from build123d import *

# Parameters (mm, degrees)
BOSS_EXTRUDE1_DEPTH  = 12
SKETCH2_R            = 1.6
CUT_EXTRUDE1_DEPTH   = 12
SKETCH3_R            = 3
CUT_EXTRUDE2_DEPTH   = 2
BOSS_EXTRUDE2_DEPTH  = 2
MIRROR2_COPY_1_DEPTH = 2
SKETCH5_W            = 40
SKETCH5_H            = 1
CUT_EXTRUDE3_DEPTH   = 20


with BuildPart() as part:
    # Sketch1 → Boss-Extrude1 (new body)
    with BuildSketch(Plane(origin=(0, 0, 0), x_dir=(1, 0, 0), z_dir=(0, 1, 0))):
        with BuildLine():
            Line((13, 0), (20, 0))
            Line((20, 0), (20, 5))
            Line((20, 5), (12, 5))
            ThreePointArc((12, 5), (12.747548784, 2.549509757), (13, 0))
        make_face()
        with BuildLine():
            Line((8, 0), (13, 0))
            ThreePointArc((13, 0), (12.747548784, 2.549509757), (12, 5))
            Line((12, 5), (6.244997998, 5))
            ThreePointArc((6.244997998, 5), (7.548509256, 2.649529771), (8, 0))
        make_face()
        with BuildLine():
            ThreePointArc((-12, 5), (-12.747548784, 2.549509757), (-13, 0))
            Line((-13, 0), (-8, 0))
            ThreePointArc((-8, 0), (-7.548509256, 2.649529771), (-6.244997998, 5))
            Line((-6.244997998, 5), (-12, 5))
        make_face()
        with BuildLine():
            Line((6.244997998, 5), (12, 5))
            ThreePointArc((12, 5), (0, 13), (-12, 5))
            Line((-12, 5), (-6.244997998, 5))
            ThreePointArc((-6.244997998, 5), (0, 8), (6.244997998, 5))
        make_face()
        with BuildLine():
            Line((-20, 0), (-13, 0))
            ThreePointArc((-13, 0), (-12.747548784, 2.549509757), (-12, 5))
            Line((-12, 5), (-20, 5))
            Line((-20, 5), (-20, 0))
        make_face()
    extrude(amount=BOSS_EXTRUDE1_DEPTH)

    # Sketch2 → Cut-Extrude1 (cut)
    with BuildSketch(Plane(origin=(0, 0, -5), x_dir=(-1, 0, 0), z_dir=(0, 0, -1))):
        with Locations((16, 6)):
            Circle(SKETCH2_R)
        with Locations((-16, 6)):
            Circle(SKETCH2_R)
    extrude(amount=-CUT_EXTRUDE1_DEPTH, mode=Mode.SUBTRACT)

    # Sketch3 → Cut-Extrude2 (cut)
    with BuildSketch(Plane(origin=(0, 0, -5), x_dir=(-1, 0, 0), z_dir=(0, 0, -1))):
        with Locations((16, 6)):
            Circle(SKETCH3_R)
        with Locations((-16, 6)):
            Circle(SKETCH3_R)
    extrude(amount=-CUT_EXTRUDE2_DEPTH, mode=Mode.SUBTRACT)

    # Sketch4 → Boss-Extrude2 (add)
    with BuildSketch(Plane(origin=(0, 12, 0), x_dir=(1, 0, 0), z_dir=(0, 1, 0))):
        Polygon((-20, 5), (-5.505882353, 11.776470588), (-3.437353346, 7.352116879), (-12, 5), align=None)
    boss_extrude2 = extrude(amount=-BOSS_EXTRUDE2_DEPTH)

    # Mirror1: Boss-Extrude2 across plane
    add(boss_extrude2.mirror(Plane(origin=(0, 0, 0), x_dir=(0, 0, 1), z_dir=(1, 0, 0))))

    # Mirror2: Boss-Extrude2 across plane
    add(boss_extrude2.mirror(Plane.ZX.offset(6)))

    # Mirror2 copy 1 sketch → Mirror2 copy 1 (add)
    with BuildSketch(Plane(origin=(0, 0, 0), x_dir=(-1, 0, 0), z_dir=(0, -1, 0))):
        Polygon((-20, 5), (-5.505882353, 11.776470588), (-3.437353346, 7.352116879), (-12, 5), align=None)
    extrude(amount=-MIRROR2_COPY_1_DEPTH)

    # Chamfer1
    # the kernel refuses this chamfer: 5 mm, written as the material it adds along each edge
    with BuildSketch(Plane(origin=(-12, 2, -5), x_dir=(0.5282334615554308, 0, -0.8490991756521539), z_dir=(0, 1, 0))) as chamfer1_piece_1_section:
        with BuildLine():
            Line((3.55102746, 0), (-2.413771098, 3.712725473))
            Line((-2.413771098, 3.712725473), (-2.498681015, 3.659902127))
            ThreePointArc((-2.498681015, 3.659902127), (-1.254288539, 1.826872841), (-0.084909918, -0.052823346))
            Line((-0.084909918, -0.052823346), (0.016102351, -0.098695057))
            ThreePointArc((0.016102351, -0.098695057), (1.773886736, 0.065687387), (3.541120329, -0.099508034))
            Line((3.541120329, -0.099508034), (3.55102746, 0))
        make_face()
    chamfer1_piece_1 = extrude(amount=8, mode=Mode.PRIVATE)
    chamfer1_piece_1 = chamfer1_piece_1 - Plane(origin=(-16, 6, -6.086552006), x_dir=(-1, 0, 0), z_dir=(0, 0, -1)) * Cylinder(3, 31, mode=Mode.PRIVATE)
    add(chamfer1_piece_1)
    with BuildSketch(Plane(origin=(12, 2, -5), x_dir=(0.9998009840016291, 0, 0.01994974659924107), z_dir=(0, 1, 0))) as chamfer1_piece_2_section:
        with BuildLine():
            Line((4.428388121, 0), (-1.935550186, 2.977153255))
            Line((-1.935550186, 2.977153255), (-2.013576875, 2.914608585))
            ThreePointArc((-2.013576875, 2.914608585), (-0.911816487, 1.523016637), (-0.091522024, -0.040295399))
            Line((-0.091522024, -0.040295399), (0.001994975, -0.099980098))
            ThreePointArc((0.001994975, -0.099980098), (2.215307803, -0.055816279), (4.430383096, -0.099980098))
            Line((4.430383096, -0.099980098), (4.428388121, 0))
        make_face()
    chamfer1_piece_2 = extrude(amount=8, mode=Mode.PRIVATE)
    chamfer1_piece_2 = chamfer1_piece_2 - Plane(origin=(16, 6, -6.086550713), x_dir=(-1, 0, 0), z_dir=(0, 0, -1)) * Cylinder(3, 34, mode=Mode.PRIVATE)
    add(chamfer1_piece_2)

    # Sketch5 → Cut-Extrude3 (cut)
    with BuildSketch(Plane.XZ):
        with Locations((0, -0.5)):
            Rectangle(SKETCH5_W, SKETCH5_H)
    extrude(amount=-CUT_EXTRUDE3_DEPTH, mode=Mode.SUBTRACT)


solid = part.part
The listing builds one solid part. Answer for the finished solid, in the listing's coordinates (mm). A direction names the side the tool comes from. Give positions to 0.01 mm unless a question says otherwise; leave off trailing zeros. Loops run counter-clockwise (first coordinate to the right, second up) from the corner with the lowest first, then second, coordinate; pieces in that order, holes last. Notation, with made-up numbers: M 42.5,42 L 54.5,42 A27 cw 54.5,65 Z; hole C 66,-36 d8. An arc over 180 degrees is marked long. Answer as CSV lines item,"result".
Item 1: Which of the six approach directions +Z, -Z, +X, -X, +Y, -Y give full straight-line access (tool end or side, diameter ignored) to faces 1 (the flat face through (-13, 10, -7)), 2 (the flat face through (-17.3, 4.7, -3)), 3 (the flat face through (19.4, 5.9, -5)), 4 (the flat face through (-20, 6, -3))?
Values follow:
face 1,"-Z, -X"
face 2,"-Z"
face 3,"-Z, +X"
face 4,"+Z, -Z, -X, +Y, -Y"
Item 2: The part is cut by section C-C (x = 7). Give the vertices of the cut face in (y, z), and give its area (3 significant figures).
Values follow:
outline,"M 0,-11.08 L 2,-11.08 L 2,-10.95 L 10,-10.95 L 10,-11.08 L 12,-11.08 L 12,-3.87 L 0,-3.87 Z"
area,"85.5 mm^2"
Item 3: The part is cut by section D-D (y = 4). Give the vertices of the cut face in (x, z) (3 decimals).
Values follow:
outline,"M -20,-5 L -18.236,-5 L -18.236,-3 L -13.764,-3 L -13.764,-6.223 L -10.304,-7.927 A13 ccw 10.304,-7.927 L 13.764,-6.223 L 13.764,-3 L 18.236,-3 L 18.236,-5 L 20,-5 L 20,-1 L 7.937,-1 A8 cw -7.937,-1 L -20,-1 Z"
Item 4: Given pin 1 Ø6 at (x, y) = (-0.5, 8.5) entering from +Z; pin 2 Ø3.5 at (x, y) = (-16, 6) entering from -Z; pin 3 Ø4 at (x, y) = (-19, 6) entering from -Z, each flat-ended and moving along its own axis, determine where each tip first touches the part or whether it passes through.
Values follow:
pin 1,"stops at z = -7.19"
pin 2,"stops at z = -3"
pin 3,"stops at z = -5"
Item 5: The part is cut by section A-A (y = 6). Give the vertices of the cut face in (x, z) (3 decimals).
Values follow:
outline,"M -20,-5 L -19,-5 L -19,-3 L -17.6,-3 L -17.6,-1 L -20,-1 Z; M -14.4,-3 L -13,-3 L -13,-6.599 L -10.304,-7.927 A13 ccw 10.304,-7.927 L 13,-6.599 L 13,-3 L 14.4,-3 L 14.4,-1 L 7.937,-1 A8 cw -7.937,-1 L -14.4,-1 Z; M 17.6,-3 L 19,-3 L 19,-5 L 20,-5 L 20,-1 L 17.6,-1 Z"
Item 6: Straight lines are drawn through the part: line 1 along Y through (x, z) = (16, -1.6); line 2 along Y through (x, z) = (-16, -4.8); line 3 along X through (y, z) = (6, -4.2). For each, find the intervals that lie inside material, in ascending order. Write a range as [from, to].
Values follow:
line 1,"y = [0, 4.4], [7.6, 12]"
line 2,"y = [0, 3], [9, 12]"
line 3,"x = [-20, -19], [-13, -6.81], [6.81, 13], [19, 20]"
Item 7: The part is cut by section B-B (z = -11). Give the vertices of the cut face in (x, y), and give its area (3 significant figures).
Values follow:
outline,"M -7.17,0 L 7.17,0 L 7.17,2 L 6.93,2 L 6.93,10 L 7.17,10 L 7.17,12 L -7.17,12 L -7.17,10 L -6.93,10 L -6.93,2 L -7.17,2 Z"
area,"168 mm^2"
